Autodesk Inventor part; units mm, degrees
ref_plane "to_rivet_XY" through (0, -4.4704, 0) normal (0, 1, 0) x (1, 0, 0)
ref_plane "to_rivet_YZ" through (0, -4.4704, 0) normal (1, 0, 0) x (0, 0, -1)
ref_plane "to_rivet_ZX" through (0, -4.4704, 0) normal (0, 0, -1) x (0, 1, 0)
sketch "Sketch_1" plane through (0, 0, 0) normal (0, 0, 1) x (1, 0, 0)
  line L0 (0, -10.8204) -> (0, -4.4704)
  line L1 (0, -4.4704) -> (9.2111, -4.4704)
  arc A0 (9.2111, -4.4704) -> (10.6049, -3.6564) centre (9.2111, -2.8702) ccw
  arc A1 (16.8656, 0) -> (10.6049, -3.6564) centre (16.8656, -7.1882) ccw
  line L2 (16.8656, 0) -> (25.4, 0)
  line L3 (25.4, 0) -> (25.4, -6.35)
  line L4 (25.4, -6.35) -> (17.3228, -6.35)
  arc A2 (17.3228, -6.35) -> (13.056, -8.1128) centre (17.3228, -12.3952) ccw
  line L5 (13.056, -8.1128) -> (10.8068, -10.3538)
  arc A3 (9.6774, -10.8204) -> (10.8068, -10.3538) centre (9.6774, -9.2202) ccw
  line L6 (9.6774, -10.8204) -> (0, -10.8204)
  line L7 (0, -10.8204) -> (0, -4.4704)
revolve "Revolution1" add sketch "Sketch_1" angle 360 about axis through (0, -10.8204, 0) along (0, -1, 0)
sketch "Sketch_2" plane through (0, 0, 0) normal (0, 1, 0) x (-1, 0, 0)
  line L0 (46.0375, 0) -> (25.4, 0)
  arc A0 (-25.4, 0) -> (25.4, 0) centre (0, 0) ccw
  line L1 (-25.4, 0) -> (-46.0375, 0)
  line L2 (-46.0375, 0) -> (-46.0375, -22.225)
  arc A1 (-46.0375, -22.225) -> (-36.5125, -31.75) centre (-36.5125, -22.225) ccw
  line L3 (-36.5125, -31.75) -> (36.5125, -31.75)
  arc A2 (36.5125, -31.75) -> (46.0375, -22.225) centre (36.5125, -22.225) ccw
  line L4 (46.0375, -22.225) -> (46.0375, 0)
  arc A3 (-35.7188, -26.543) -> (-35.7188, -17.907) centre (-35.7187, -22.225) ccw
  line L5 (-35.7188, -17.907) -> (-38.8937, -17.907)
  arc A4 (-38.8937, -17.907) -> (-38.8937, -26.543) centre (-38.8938, -22.225) ccw
  line L6 (-38.8937, -26.543) -> (-35.7188, -26.543)
  arc A5 (38.8937, -26.543) -> (38.8937, -17.907) centre (38.8938, -22.225) ccw
  line L7 (38.8937, -17.907) -> (35.7188, -17.907)
  arc A6 (35.7188, -17.907) -> (35.7188, -26.543) centre (35.7187, -22.225) ccw
  line L8 (35.7188, -26.543) -> (38.8937, -26.543)
extrude "Extrusion1" add sketch "Sketch_2" against normal blind 6.35
sketch "Sketch_3" plane through (0, 0, 0) normal (0, 1, 0) x (-1, 0, 0)
  line L0 (46.0375, 0) -> (46.0375, 22.225)
  arc A0 (46.0375, 22.225) -> (36.5125, 31.75) centre (36.5125, 22.225) ccw
  line L1 (36.5125, 31.75) -> (-36.5125, 31.75)
  arc A1 (-36.5125, 31.75) -> (-46.0375, 22.225) centre (-36.5125, 22.225) ccw
  line L2 (-46.0375, 22.225) -> (-46.0375, 0)
  line L3 (-46.0375, 0) -> (-25.4, 0)
  arc A2 (25.4, 0) -> (-25.4, 0) centre (0, 0) ccw
  line L4 (25.4, 0) -> (46.0375, 0)
  arc A3 (-35.7188, 17.907) -> (-35.7188, 26.543) centre (-35.7187, 22.225) ccw
  line L5 (-35.7188, 26.543) -> (-38.8937, 26.543)
  arc A4 (-38.8937, 26.543) -> (-38.8937, 17.907) centre (-38.8938, 22.225) ccw
  line L6 (-38.8937, 17.907) -> (-35.7188, 17.907)
  arc A5 (38.8937, 17.907) -> (38.8937, 26.543) centre (38.8938, 22.225) ccw
  line L7 (38.8937, 26.543) -> (35.7188, 26.543)
  arc A6 (35.7188, 26.543) -> (35.7188, 17.907) centre (35.7187, 22.225) ccw
  line L8 (35.7188, 17.907) -> (38.8937, 17.907)
extrude "Extrusion2" add sketch "Sketch_3" against normal blind 6.35
ref_plane "to_rivet_XY" through (0, -4.4704, 0) normal (0, 1, 0) x (1, 0, 0)
ref_plane "to_rivet_YZ" through (0, -4.4704, 0) normal (1, 0, 0) x (0, 0, -1)
ref_plane "to_rivet_ZX" through (0, -4.4704, 0) normal (0, 0, -1) x (0, 1, 0)
ref_plane "to_upper_race_XY" through (0, -6.35, 0) normal (0, 1, 0) x (1, 0, 0)
ref_plane "to_upper_race_YZ" through (0, -6.35, 0) normal (1, 0, 0) x (0, 0, -1)
ref_plane "to_upper_race_ZX" through (0, -6.35, 0) normal (0, 0, -1) x (0, 1, 0)
ref_plane "top_plate_XY" through (0, 0, 0) normal (0, -1, 0) x (1, 0, 0)
ref_plane "top_plate_YZ" through (0, 0, 0) normal (1, 0, 0) x (0, 0, 1)
ref_plane "top_plate_ZX" through (0, 0, 0) normal (0, 0, 1) x (0, -1, 0)
properties part number "2SS-TP"
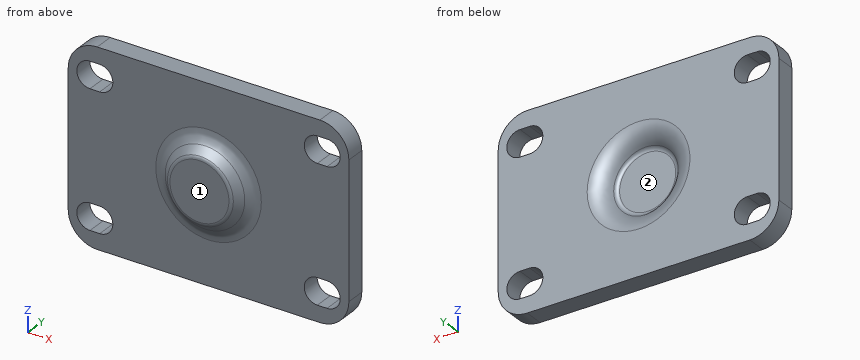
Read the model definition and answer for the solid it produces. Units are mm, in the model's axes. Face numbers are marked on the shaded views. Coordinates: 2 decimals unless noted, no trailing zeros. Write each loop counter-clockwise with the first axis right and the second up, starting at its lowest first coordinate (ties: lowest second). Pieces come first, ordered by that corner, then holes. Notation, with made-up numbers: (36.25, 53) - (53.25, 53) arc R8 ccw to (53.25, 60) - close; hole circle Ø11 at (48.5, 32.5). An arc over 180 degrees is marked (long way). Answer as a JSON object with one key per item and string values. Group by question number.
1. A cutting plane is placed at D-D (z = -21). Determine the outline of the cut face in (x, y).
2. Each of these flat-tipped pins is pushed along its axis until it touches: P1, Ø1.6, axis at x = 38, y = -3.5, coming from the +Z side; P2, Ø4, axis at x = 12, z = 4, coming from the -Y side; P3, Ø1.5, axis at x = 2.5, z = -5, coming from the +Y side. Where does it stop, or does it pass through?
3. A cutting plane is placed at C-C (y = -2). Give the number of separate pieces and of enclosed holes in the cut face, plus the area to 3 significant figures.
4. A cutting plane is placed at B-B (z = 0). Determine the outline of the cut face in (x, y).
5. A cutting plane is placed at A-A (x = 0). Determine the outline of the cut face in (y, z).
6. The mould has two halves that part along Z. Classify the marked faces 1 and 2: +Z half, -Z half, draft (parallel to the pull), parting line (faces both ways), or undercut.
7. Consider L1, parallel to Y at x = -6, z = -1; L2, parallel to Y at x = -24, z = -25; L3, parallel to Z at x = -7.5, y = -8. Determine where each line is inside the solid, lowest interval first. Write a range as [from, to].
Worked out:
{
 "1": {"outline": "(-46.04, -6.35) - (-43.03, -6.35) - (-43.03, 0) - (-46.04, 0) - close; (-31.58, -6.35) - (31.58, -6.35) - (31.58, 0) - (-31.58, 0) - close; (43.03, -6.35) - (46.04, -6.35) - (46.04, 0) - (43.03, 0) - close"},
 "2": {"P1": "stops at z = 31.73", "P2": "stops at y = -10.49", "P3": "stops at y = -4.47"},
 "3": {"separate pieces": "1", "enclosed holes": "5", "area": "4,980 mm²"},
 "4": {"outline": "(-46.04, -6.35) - (-17.32, -6.35) arc R6.05 cw to (-13.06, -8.11) - (-10.81, -10.35) arc R1.6 ccw to (-9.68, -10.82) - (9.68, -10.82) arc R1.6 ccw to (10.81, -10.35) - (13.06, -8.11) arc R6.05 cw to (17.32, -6.35) - (46.04, -6.35) - (46.04, 0) - (16.87, 0) arc R7.19 ccw to (10.6, -3.66) arc R1.6 cw to (9.21, -4.47) - (-9.21, -4.47) arc R1.6 cw to (-10.6, -3.66) arc R7.19 ccw to (-16.87, 0) - (-46.04, 0) - close"},
 "5": {"outline": "(-10.82, -9.68) arc R1.6 ccw to (-10.35, -10.81) - (-8.11, -13.06) arc R6.05 cw to (-6.35, -17.32) - (-6.35, -31.75) - (0, -31.75) - (0, -16.87) arc R7.19 ccw to (-3.66, -10.6) arc R1.6 cw to (-4.47, -9.21) - (-4.47, 9.21) arc R1.6 cw to (-3.66, 10.6) arc R7.19 ccw to (0, 16.87) - (0, 31.75) - (-6.35, 31.75) - (-6.35, 17.32) arc R6.05 cw to (-8.11, 13.06) - (-10.35, 10.81) arc R1.6 ccw to (-10.82, 9.68) - close"},
 "6": {"face 1": "draft", "face 2": "undercut"},
 "7": {"L1": "y = [-10.82, -4.47]", "L2": "y = [-6.35, 0]", "L3": "z = [-10.83, 10.83]"}
}
